The model under review builds one solid part; all positions refer to its coordinate system, in mm. A direction names the side the tool comes from. Round coordinates to 2 decimals unless told otherwise and drop trailing zeros. Loops run counter-clockwise (first coordinate to the right, second up) from the corner with the lowest first, then second, coordinate; pieces in that order, holes last. Notation, with made-up numbers: (11.25, -19.5) - (51.25, -19.5) arc R28 cw to (51.25, -0.5) - close; hole circle Ø5 at (45, -39.5). An arc over 180 degrees is marked (long way). Answer as CSV lines item,"result".
from build123d import *

# Parameters (mm, degrees)
BOSS_EXTRUDE1_DEPTH = 100
SKETCH2_R           = 2.75
CUT_EXTRUDE1_DEPTH  = 132.314063663
SKETCH3_R           = 5
CUT_EXTRUDE2_DEPTH  = 2
CUT_EXTRUDE3_DEPTH  = 4
FILLET3_R           = 3
FILLET6_R           = 2


with BuildPart() as part:
    # Sketch1 → Boss-Extrude1 (new body)
    with BuildSketch(Plane(origin=(0, 0, 0), x_dir=(1, 0, 0), z_dir=(0, 1, 0))):
        Polygon((-16.010741182, -8), (-13.18496009, -5), (-10, -8), (-10, -24), (-13.18496009, -27), (-16.010741182, -24), (-18, -24), (-18, -32), (-10, -32), (-0.5326227, -32), (9.496769329, -55.62776694), (40.799639873, -55.62776694), (64.412226021, 0), (58.980424134, 0), (37.490212067, -50.62776694), (21.490212067, -50.62776694), (0, 0), (-10, 0), (-18, 0), (-18, -8), align=None)
    extrude(amount=BOSS_EXTRUDE1_DEPTH)

    # Sketch2 → Cut-Extrude1 (cut, through all)
    with BuildSketch(Plane(origin=(0, 0, 0), x_dir=(-1, 0, 0), z_dir=(0, 0, -1))):
        with Locations((11.592480045, 50)):
            Circle(SKETCH2_R)
    extrude(amount=-CUT_EXTRUDE1_DEPTH, mode=Mode.SUBTRACT)

    # Sketch3 → Cut-Extrude2 (cut)
    with BuildSketch(Plane(origin=(0, 0, 0), x_dir=(-1, 0, 0), z_dir=(0, 0, -1))):
        with Locations((11.592480045, 50)):
            Circle(SKETCH3_R)
    extrude(amount=-CUT_EXTRUDE2_DEPTH, mode=Mode.SUBTRACT)

    # Sketch4 → Cut-Extrude3 (cut)
    with BuildSketch(Plane.XY.offset(32)):
        Polygon((-6.792480045, 47.228718708), (-6.792480045, 52.771281292), (-11.592480045, 55.542562584), (-16.392480045, 52.771281292), (-16.392480045, 47.228718708), (-11.592480045, 44.457437416), align=None)
    extrude(amount=-CUT_EXTRUDE3_DEPTH, mode=Mode.SUBTRACT)

    # Fillet3
    # the kernel refuses this fillet: 3 mm, written as the material it adds along each edge
    with BuildSketch(Plane(origin=(21.490212067, 0, 50.62776694), x_dir=(1, 0, 0), z_dir=(0, 1, 0)), Plane(origin=(37.490212067, 0, 50.62776694), x_dir=(0.39073112848927616, 0, -0.9205048534524394), z_dir=(0, 1, 0)), Plane(origin=(-0.5326227, 0, 32), x_dir=(-1, 0, 0), z_dir=(0, 1, 0))) as fillet3_piece_1:
        with BuildLine():
            CenterArc((FILLET3_R * 0.661885561196, FILLET3_R), FILLET3_R, 203, 67)
            Line((-FILLET3_R * 0.258619292257, FILLET3_R * 0.609268871511), (0, 0))
            Line((0, 0), (FILLET3_R * 0.661885561196, 0))
        make_face()
    extrude(amount=100)
    # the kernel refuses this fillet: 3 mm, written as the material it takes off along each edge
    with BuildSketch(Plane(origin=(0, -4.964141709, 0), x_dir=(0.39073112848927805, 0, 0.9205048534524385), z_dir=(0, 1, 0)), Plane(origin=(58.980424134, -4.964141709, 0), x_dir=(1, 0, 0), z_dir=(0, 1, 0)), Plane(origin=(40.799639873, -4.964141709, 55.62776694), x_dir=(-1, 0, 0), z_dir=(0, 1, 0)), Plane(origin=(9.496769329, -4.964141709, 55.62776694), x_dir=(-0.3907311284892769, 0, -0.920504853452439), z_dir=(0, 1, 0))) as fillet3_2_piece_1:
        with BuildLine():
            CenterArc((FILLET3_R * 0.661885561196, -FILLET3_R), FILLET3_R, 90, 67)
            Line((-FILLET3_R * 0.258619292257, -FILLET3_R * 0.609268871511), (0, 0))
            Line((0, 0), (FILLET3_R * 0.661885561196, 0))
        make_face()
    extrude(amount=109.928283418, mode=Mode.SUBTRACT)
    with BuildSketch(Plane(origin=(64.412226021, -11.331263952, 0), x_dir=(-0.3907311284892779, 0, 0.9205048534524386), z_dir=(0, 1, 0))) as fillet3_2_piece_2:
        with BuildLine():
            CenterArc((FILLET3_R * 1.51083519361, -FILLET3_R), FILLET3_R, 90, 113)
            Line((FILLET3_R * 0.590330340162, -FILLET3_R * 1.39073112849), (0, 0))
            Line((0, 0), (FILLET3_R * 1.51083519361, 0))
        make_face()
    extrude(amount=122.662527904, mode=Mode.SUBTRACT)

    # Fillet6
    fillet6_edges = [part.edges().sort_by_distance(p)[0] for p in [
        (-11.592480045, 100, 6.5),
        (-10, 100, 16),
        (-11.592480045, 100, 25.5),
        (-14.597850636, 100, 25.5),
        (-17.005370591, 100, 24),
        (-17.005370591, 0, 24),
        (-14.597850636, 0, 25.5),
        (-11.592480045, 0, 25.5),
        (-10, 0, 16),
        (-11.592480045, 0, 6.5),
        (-14.597850636, 0, 6.5),
        (-17.005370591, 0, 8),
        (-17.005370591, 100, 8),
        (-14.597850636, 100, 6.5),
    ]]
    fillet(fillet6_edges, radius=FILLET6_R)


solid = part.part
1. Take a section at A-A (y = 84.5). State the section outline as (x, z) points.
Numbers:
outline,"(-18, 0) - (-1.99, 0) arc R3 ccw to (0.78, 1.83) - (20.71, 48.8) arc R3 cw to (23.48, 50.63) - (35.5, 50.63) arc R3 cw to (38.27, 48.8) - (58.2, 1.83) arc R3 ccw to (60.42, 0.05) arc R3 ccw to (62.64, 4.17) - (41.58, 53.8) arc R3 ccw to (38.81, 55.63) - (11.48, 55.63) arc R3 ccw to (8.72, 53.8) - (0.24, 33.83) arc R3 cw to (-2.52, 32) - (-18, 32) - (-18, 24) - (-16.01, 24) - (-13.18, 27) - (-10, 24) - (-10, 8) - (-13.18, 5) - (-16.01, 8) - (-18, 8) - close"
2. Take a section at D-D (y = 50). State how many separate pieces and enclosed holes the cut face has, plus the area to 3 significant figures.
Numbers:
separate pieces,"3"
enclosed holes,"0"
area,"1,230 mm²"
3. Tool access review of faces 1 (the face through (-14.787, 0.57, 5.824)), 2 (the face through (-14.28, 54.216, 0.986)), 3 (the face through (-6.792, 50, 30)), 4 (the face through (-11.615, 74.801, 6.479)), 5 (the face through (10.885, 49.3, 25.643)): name each direction out of +Z, -Z, +X, -X, +Y, -Y from which nothing blocks a thin tool from reaching the whole face with its end or side.
Numbers:
face 1,"-Y"
face 2,"-Z"
face 3,"+Z"
face 4,"+Y, -Y"
face 5,"-Z, +Y, -Y"
4. Take a section at C-C (x = 34). State the section outline as (y, z) points.
Numbers:
outline,"(0, 50.63) - (100, 50.63) - (100, 55.63) - (0, 55.63) - close"
5. Draft analysis for pull direction Z (two halves, no side actions). For faces 6 (the face through (-11.615, 24.559, 6.479)), 7 (the face through (4.42, 49.3, 43.67)), 8 (the face through (11, 100, 30)), 9 (the face through (-14.85, 0.57, 26.11)), state which applies: +Z half, -Z half, draft (parallel to the pull), parting line (faces both ways), or undercut.
Numbers:
face 6,"undercut"
face 7,"+Z half"
face 8,"draft"
face 9,"undercut"
6. Wall thickness on probe 1 along Z at (x, y) = (-3.5, 40); probe 2 along Z at (x, y) = (27.5, 41.5); probe 3 along Z at (x, y) = (-13, 12): over which ranges is each line inside the solid? List them lowest first.
Numbers:
probe 1,"z = 0 to 32"
probe 2,"z = 50.63 to 55.63"
probe 3,"z = 0 to 5.17, 26.83 to 32"
7. Clearance check with flat-ended pins moving along their axes: pin 1 (13 mm diameter, centred on x = 29.5, y = 36.5, fed in from -Z); pin 2 (1.6 mm diameter, centred on x = -17, y = 49.5, fed in from +Z); pin 3 (10 mm diameter, centred on y = 51, z = 8.5, fed in from -X); pin 4 (5 mm diameter, centred on x = -12.5, y = 48, fed in from +Z). State where each tip first meets the part, or that it passes through.
Numbers:
pin 1,"stops at z = 50.59"
pin 2,"stops at z = 32"
pin 3,"stops at x = -18"
pin 4,"stops at z = 28"
8. Take a section at B-B (z = 40). State the section outline as (x, y) points, plus the area to 3 significant figures.
Numbers:
outline,"(2.86, 0) - (16.98, 0) - (16.98, 100) - (2.86, 100) - close; (42, 0) - (47.43, 0) - (47.43, 100) - (42, 100) - close"
area,"1,950 mm²"
